from build123d import *

# Parameters (mm, degrees)
F1_DEPTH  = 127
F2_SIZE   = 20
F3_DEPTH  = 100.7419452071
F4_W      = 73.9247704289
F4_H      = 28.8404997019
F5_DEPTH  = 227.7429452071
F10_DEPTH = 112.4425134991


# Not quite as in the source:
# - the program builds the solid bodies; features that only make, move or delete a surface that nothing else refers to are left out


with BuildPart() as f1:
    # F0 (on Top) → F1 (new body)
    with BuildSketch(Plane.XY):
        Polygon((-44.9766053996, -25.9672552347), (0, -51.9345104694), (44.9766053996, -25.9672552347), (44.9766053996, 25.9672552347), (0, 51.9345104694), (-44.9766053996, 25.9672552347), align=None)
    extrude(amount=F1_DEPTH)

    # F2
    f2_edges = [f1.edges().sort_by_distance(p)[0] for p in [
        (-44.976605, 0, 127),
        (-22.488303, 38.950883, 127),
        (22.488303, 38.950883, 127),
        (44.976605, 0, 127),
        (22.488303, -38.950883, 127),
        (-22.488303, -38.950883, 127),
    ]]
    chamfer(f2_edges, length=F2_SIZE)

    # F3 (add): a face of the model
    f3_faces = [f1.faces().sort_by_distance(p)[0] for p in [
        (0, 0, 127),
    ]]
    extrude(f3_faces, amount=F3_DEPTH)

    # F4 (on face) → F5 (cut, through all)
    with BuildSketch(Plane.XY.offset(227.7419452071)):
        with Locations((11.9857798148, 0)):
            Rectangle(F4_W, F4_H)
    extrude(amount=-F5_DEPTH, mode=Mode.SUBTRACT)

    # F8 (on face) → F10 (cut, through all)
    with BuildSketch(Plane(origin=(-22.4883026998, -38.9508828521, 0), x_dir=(0.8660254038, -0.5, 0), z_dir=(-0.5, -0.8660254038, 0))):
        with BuildLine():
            add(Edge.make_bspline(
                [(0, 67.8614079952), (35.7205863144, 67.8614079952), (17.8602931572, 91.3859009743), (0, 114.9103939533), (-17.8602931572, 91.3859009743), (-35.7205863144, 67.8614079952), (0, 67.8614079952)],
                knots=[4.7123889804, 4.7123889804, 4.7123889804, 6.8067840828, 6.8067840828, 8.9011791852, 8.9011791852, 10.9955742876, 10.9955742876, 10.9955742876], degree=2, weights=[1, 0.5, 1, 0.5, 1, 0.5, 1]))
        make_face()
    extrude(amount=-F10_DEPTH, mode=Mode.SUBTRACT)


solid = f1.part
The listing builds one solid part. Answer for the finished solid, in the listing's coordinates (mm). A direction names the side the tool comes from. Coordinates: 2 decimals unless noted, no trailing zeros. Loops run counter-clockwise (first coordinate to the right, second up) from the corner with the lowest first, then second, coordinate; pieces in that order, holes last. Notation, with made-up numbers: (22.5, -22.75) -> (53.5, -22.75) arc R8 ccw to (53.5, -16.75) -> close; hole circle Ø2 at (27.25, 40.5). An arc over 180 degrees is marked (long way). Answer in a Markdown table with one row per item. Add a question column.
1. For faces 5 (the flat face through (12.313, -21.731, 176.666)), 6 (the flat face through (-12.66, -21.53, 176.67)), 7 (the flat face through (12.66, 21.53, 176.67)), 8 (the flat face through (-24.977, 0, 64)), determine the directions among +Z, -Z, +X, -X, +Y, -Y from which every point of the face is accessible in a straight line to the end or side of a thin tool.
2. The part is cut by section A-A, the plane z = 193.5. Write down the section's boundary in (x, y), then the cut area to 3 significant figures.
3. The part is cut by section C-C, the plane x = -13. Count the separate pieces of the cut face and the enclosed holes in it, then the cut area to 3 significant figures.
4. The part is cut by section D-D, the plane z = 112. Write down the section's boundary in (x, y), then the cut area to 3 significant figures.
5. Consider line 1 (Z direction, x = 4.5, y = 21); line 2 (Y direction, x = 20, z = 15); line 3 (Y direction, x = 3.5, z = 150.5). Determine where each line is inside the solid, lowest interval first. Write a range as [from, to].
6. The part is cut by section B-B, the plane z = 14.5. Write down the section's boundary in (x, y).
7. Determine the mould class of faces 1 (the flat face through (-44.977, 0, 53)), 2 (the flat face through (2, 14.42, 115)), 3 (the flat face through (-12.313, 21.731, 176.666)), 4 (the flat face through (17.1, -30.4, 117.1)) for opening direction Y: +Y half, -Y half, draft (parallel to the pull), parting line (faces both ways), or undercut.
8. Flat-ended cylindrical pins translate along their axes: P1, Ø2, axis at y = -33, z = 55, coming from the -X side; P2, Ø10, axis at x = 17.5, y = -28.5, coming from the +Z side; P3, Ø6, axis at y = 8.5, z = 51, coming from the +X side; P4, Ø1.5, axis at x = 0.5, y = 12.5, coming from the -Z side. Find the tip coordinate at first contact, or state that the pin passes through.
Answer below:
| question | item | result |
|---|---|---|
| 1 | face 5 | +Z, +X, -Y |
| 1 | face 6 | +Z, -X, -Y |
| 1 | face 7 | +Z, +X, +Y |
| 1 | face 8 | +Z, -Z, +X |
| 2 | outline | (-24.98, -14.42) -> (0, -28.84) -> (24.98, -14.42) -> close; (-24.98, 14.42) -> (24.98, 14.42) -> (0, 28.84) -> close |
| 2 | area | 720 mm2 |
| 3 | separate pieces | 3 |
| 3 | enclosed holes | 0 |
| 3 | area | 7,610 mm2 |
| 4 | outline | (-39.98, -23.08) -> (0, -46.16) -> (39.98, -23.08) -> (39.98, -14.42) -> (-24.98, -14.42) -> (-24.98, 14.42) -> (39.98, 14.42) -> (39.98, 23.08) -> (0, 46.16) -> (-39.98, 23.08) -> close |
| 4 | area | 3,660 mm2 |
| 5 | line 1 | [0, 68.69], [98.4, 227.74] |
| 5 | line 2 | [-40.39, -14.42], [14.42, 40.39] |
| 5 | line 3 | [-26.82, -14.42], [14.42, 26.82] |
| 6 | outline | (-44.98, -25.97) -> (0, -51.93) -> (44.98, -25.97) -> (44.98, -14.42) -> (-24.98, -14.42) -> (-24.98, 14.42) -> (44.98, 14.42) -> (44.98, 25.97) -> (0, 51.93) -> (-44.98, 25.97) -> close |
| 7 | face 1 | draft |
| 7 | face 2 | undercut |
| 7 | face 3 | +Y half |
| 7 | face 4 | -Y half |
| 8 | P1 | x = -34.53 |
| 8 | P2 | z = 123.54 |
| 8 | P3 | x = -24.98 |
| 8 | P4 | through |
